Model file for the job. Use its own axes, mm. A direction names the side the tool comes from. Give positions to 0.01 mm unless a question says otherwise; leave off trailing zeros. Write each loop counter-clockwise with the first axis right and the second up, starting at its lowest first coordinate (ties: lowest second). Pieces come first, ordered by that corner, then holes. Notation, with made-up numbers: (82, 42.5) - (115, 42.5) arc R5 ccw to (115, 46.5) - close; hole circle Ø5 at (-24, 57). An arc over 180 degrees is marked (long way). Use CSV: the item, a comma, the result in double quotes.
from build123d import *

# Parameters (mm, degrees)
F0_W     = 203.2
F0_H     = 127
F1_DEPTH = 127
F3_DEPTH = 76.2
F4_SIZE2 = 101.6
F4_SIZE  = 76.2
F5_R     = 5.08
F6_R     = 15.24
F7_DEPTH = 50.8
F8_R     = 12.7
F9_DEPTH = 127


with BuildPart() as f1:
    # F0 (on Front) → F1 (new body)
    with BuildSketch(Plane.XZ):
        with Locations((15.3181515634, -8.0336100439)):
            Rectangle(F0_W, F0_H)
    extrude(amount=F1_DEPTH)

    # F2 (on face) → F3 (cut)
    with BuildSketch(Plane.XZ.offset(127)):
        Polygon((-22.7818484366, -8.0336100439), (-22.7818484366, -71.5336100439), (116.9181515634, -71.5336100439), (116.9181515634, 55.4663899561), (15.3181515634, 55.4663899561), (15.3181515634, 37.2199955379), (15.3181515634, -8.0336100439), align=None)
    extrude(amount=-F3_DEPTH, mode=Mode.SUBTRACT)

    # F4
    f4_edges = [f1.edges().sort_by_distance(p)[0] for p in [
        (116.918152, -25.4, 55.46639),
    ]]
    f4_side = f1.faces().sort_by_distance((-6.453277, -52.614286, 55.46639))[0]
    chamfer(f4_edges, length=F4_SIZE, length2=F4_SIZE2, reference=f4_side)

    # F5
    f5_edges = [f1.edges().sort_by_distance(p)[0] for p in [
        (15.318152, -88.9, 55.46639),
        (-35.481848, -127, 55.46639),
        (15.318152, -127, 23.71639),
        (15.318152, -88.9, -8.03361),
        (-22.781848, -88.9, -8.03361),
        (-22.781848, -88.9, -71.53361),
        (-22.781848, -127, -39.78361),
        (-22.781848, -50.8, -39.78361),
        (-3.731848, -127, -8.03361),
        (-54.531848, -127, -71.53361),
        (-86.281848, -127, -8.03361),
        (-86.281848, -63.5, 55.46639),
        (-86.281848, -63.5, -71.53361),
        (-86.281848, 0, -8.03361),
        (-22.781848, 0, 55.46639),
        (40.718152, -25.4, 55.46639),
        (28.018152, -50.8, 55.46639),
        (47.068152, -50.8, -71.53361),
    ]]
    fillet(f5_edges, radius=F5_R)

    # F6 (on face) → F7 (cut, through all)
    with BuildSketch(Plane.XZ.offset(50.8)):
        with Locations((33.0981515634, -25.8136100439)):
            Circle(F6_R)
    extrude(amount=-F7_DEPTH, mode=Mode.SUBTRACT)

    # F8 (on face) → F9 (cut, through all)
    with BuildSketch(Plane.XY.offset(55.4663899561)):
        with Locations((-62.5347197056, -91.1505147815)):
            Circle(F8_R)
    extrude(amount=-F9_DEPTH, mode=Mode.SUBTRACT)


solid = f1.part
(1) Saw through at A-A, the plane z = -34. List the corners of the cut face in (x, y).
Checked values:
outline,"(-86.28, -121.92) arc R5.08 ccw to (-81.2, -127) - (-27.86, -127) arc R5.08 ccw to (-22.78, -121.92) - (-22.78, -55.88) arc R5.08 cw to (-17.7, -50.8) - (20.24, -50.8) - (20.24, 0) - (-81.2, 0) arc R5.08 ccw to (-86.28, -5.08) - close; (45.95, -50.8) - (107.82, -50.8) - (107.82, 0) - (45.95, 0) - close; hole circle Ø25.4 at (-62.53, -91.15)"
(2) Saw through at C-C, the plane x = 30. List the corners of the cut face in (y, z), then the cut area to 3 significant figures.
Checked values:
outline,"(-50.8, -66.45) arc R5.08 ccw to (-45.72, -71.53) - (0, -71.53) - (0, -40.74) - (-50.8, -40.74) - close; (-50.8, -10.89) - (0, -10.89) - (0, 50.39) arc R5.08 ccw to (-5.08, 55.47) - (-45.72, 55.47) arc R5.08 ccw to (-50.8, 50.39) - close"
area,"4,920 mm^2"
(3) 3-axis set-ups, long thin cutter, end or side, ignore diameter. For faces 1 (the face through (27.14, -49.27, 54.02)), 2 (the face through (-4, -87, -8.034)), 3 (the face through (-84.83, -61.81, -70.01)): which of +Z, -Z, +X, -X, +Y, -Y reach the whole face in a straight line?
Checked values:
face 1,"+Z, +X, -Y"
face 2,"-Z, +X, -Y"
face 3,"-Z, -X, +Y, -Y"
(4) Saw through at D-D, the plane x = 7.5. List the corners of the cut face in (y, z).
Checked values:
outline,"(-127, -2.95) arc R5.08 ccw to (-121.92, -8.03) - (-50.8, -8.03) - (-50.8, -66.45) arc R5.08 ccw to (-45.72, -71.53) - (0, -71.53) - (0, 50.39) arc R5.08 ccw to (-5.08, 55.47) - (-121.92, 55.47) arc R5.08 ccw to (-127, 50.39) - close"
(5) Saw through at B-B, the plane y = -96. List the corners of the cut face in (x, z).
Checked values:
outline,"(-86.28, -66.45) arc R5.08 ccw to (-81.2, -71.53) - (-74.27, -71.53) - (-74.27, 55.47) - (-81.2, 55.47) arc R5.08 ccw to (-86.28, 50.39) - close; (-50.8, -71.53) - (-27.86, -71.53) arc R5.08 ccw to (-22.78, -66.45) - (-22.78, -13.11) arc R5.08 cw to (-17.7, -8.03) - (10.24, -8.03) arc R5.08 ccw to (15.32, -2.95) - (15.32, 50.39) arc R5.08 ccw to (10.24, 55.47) - (-50.8, 55.47) - close"
(6) Wall check: probe 1 along X at (y, z) = (-73.5, 9.5); probe 2 along Y at (x, z) = (2, -14.5); probe 3 along X at (y, z) = (-120.5, -44.5). Give the ranges that are in metal, low to high. Write a range as [from, to].
Checked values:
probe 1,"x = [-86.28, 15.32]"
probe 2,"y = [-50.8, 0]"
probe 3,"x = [-86.28, -22.78]"
(7) Flat gauge pins, fed straight in: P1, Ø22.5, axis at x = -2, y = -88.5, coming from the -Z side; P2, Ø10, axis at y = -41.5, z = 33.5, coming from the +X side; P3, Ø2, axis at x = 66, z = -33, coming from the -Y side. Where does each tip first touch, or does it go through?
Checked values:
P1,"stops at z = -8.03"
P2,"stops at x = 60.94"
P3,"stops at y = -50.8"
